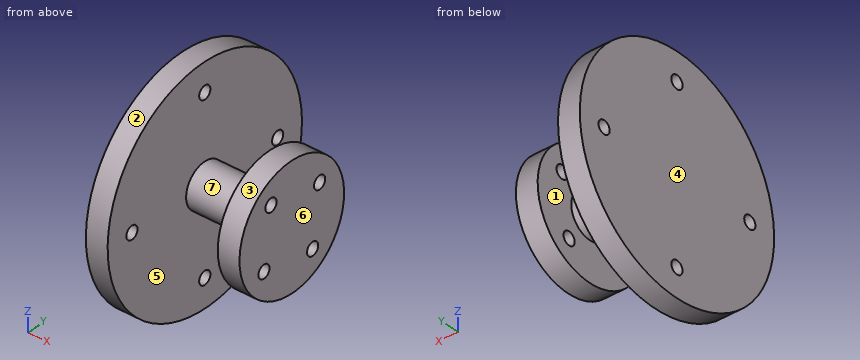
from build123d import *

# Parameters (mm, degrees)
SKETCH_2_R               = 1.5
CUT_EXTRUDE_1_DEPTH      = 45.463468151
PATTERN_CIRCULAR_1_COUNT = 4
CUT_EXTRUDE_2_REACH      = 46.463
SKETCH_3_R               = 1.5
PATTERN_CIRCULAR_2_COUNT = 4


with BuildPart() as part:
    # Sketch 1 → Revolve 1 (revolve)
    with BuildSketch(Plane.XY, mode=Mode.PRIVATE) as revolve_1_sk:
        Polygon((0, 0), (0, 26), (5, 26), (5, 5), (20, 5), (20, 14), (25, 14), (25, 0), align=None)
    revolve(revolve_1_sk.sketch.rotate(Axis((0, 0, 0), (1, 0, 0)), 90), axis=Axis((0, 0, 0), (1, 0, 0)))

    # Sketch 2 → Cut-Extrude 1 (cut, through all)
    with BuildSketch(Plane.ZY):
        with Locations((0, 19.5)):
            Circle(SKETCH_2_R)
    cut_extrude_1 = extrude(amount=-CUT_EXTRUDE_1_DEPTH, mode=Mode.SUBTRACT)

    # Pattern Circular 1: Cut-Extrude 1 ×4 about axis
    pattern_circular_1_axis = Axis((0, 0, 0), (1, 0, 0))
    for i in range(1, PATTERN_CIRCULAR_1_COUNT):
        add(cut_extrude_1.rotate(pattern_circular_1_axis, i * 360 / PATTERN_CIRCULAR_1_COUNT), mode=Mode.SUBTRACT)

    # Sketch 3 → Cut-Extrude 2 (cut, up to next)
    with BuildSketch(Plane(origin=(25, 0, 0), x_dir=(0, 0, -1), z_dir=(1, 0, 0)), mode=Mode.PRIVATE) as cut_extrude_2_sk1:
        with Locations((7.448193574, 5.569058492)):
            Circle(SKETCH_3_R)
    cut_extrude_2_tool1 = extrude(cut_extrude_2_sk1.sketch, amount=-CUT_EXTRUDE_2_REACH, mode=Mode.PRIVATE) & part.part
    cut_extrude_2 = cut_extrude_2_tool1.solids().sort_by_distance((25, 5.569058, -7.448194))[0]
    add(cut_extrude_2, mode=Mode.SUBTRACT)

    # Pattern Circular 2: Cut-Extrude 2 ×4 about axis
    pattern_circular_2_axis = Axis((0, 0, 0), (1, 0, 0))
    for i in range(1, PATTERN_CIRCULAR_2_COUNT):
        add(cut_extrude_2.rotate(pattern_circular_2_axis, i * 360 / PATTERN_CIRCULAR_2_COUNT), mode=Mode.SUBTRACT)


solid = part.part
Model file for the job. Use its own axes, mm. Face numbers are marked on the shaded views. A direction names the side the tool comes from. Round coordinates to 2 decimals unless told otherwise and drop trailing zeros. Loops run counter-clockwise (first coordinate to the right, second up) from the corner with the lowest first, then second, coordinate; pieces in that order, holes last.
1. Mould opens along X. For the marked faces 4, 5, 6 and 7 say: +X half, -X half, draft (parallel to the pull), parting line (faces both ways), or undercut.
Check values:
face 4: -X half
face 5: undercut
face 6: +X half
face 7: undercut
2. Drop flat-ended pins along their axis: P1, Ø1.8, axis at y = -5.57, z = 7.45, coming from the +X side; P2, Ø12, axis at x = 4.5, z = -15, coming from the -Y side; P3, Ø2, axis at x = 5.5, y = 1, coming from the +Z side; P4, Ø2.5, axis at y = 19.5, z = 0, coming from the +X side. Give the stop position or say it passes through.
Check values:
P1: stops at x = 5
P2: stops at y = -24.39
P3: stops at z = 26
P4: passes through
3. Band-saw the part on D-D, the plane y = -11. List the corners of the cut face in (x, z).
Check values:
outline: (0, -23.56) - (5, -23.56) - (5, 23.56) - (0, 23.56) - close; (20, -8.66) - (25, -8.66) - (25, 8.66) - (20, 8.66) - close
4. Wall check: probe 1 along Y at (x, z) = (2.25, -0.5); probe 2 along X at (y, z) = (-5.5, -10); probe 3 along X at (y, z) = (16, -2.5). Give the ranges that are in metal, low to high.
Check values:
probe 1: y = -26 to -20.91, -18.09 to 18.09, 20.91 to 26
probe 2: x = 0 to 5, 20 to 25
probe 3: x = 0 to 5
5. Tool access for the marked faces 1, 2 and 3: list every direction of +Z, -Z, +X, -X, +Y, -Y with a clear straight run to the whole face (end or side of a thin tool).
Check values:
face 1: none
face 2: +X, -X
face 3: +X
6. Band-saw the part on C-C, the plane z = 19.5. List the corners of the cut face in (x, y).
Check values:
outline: (0, -17.2) - (5, -17.2) - (5, -1.5) - (0, -1.5) - close; (0, 1.5) - (5, 1.5) - (5, 17.2) - (0, 17.2) - close
7. Band-saw the part on A-A, the plane z = 0. List the corners of the cut face in (x, y).
Check values:
outline: (0, -26) - (5, -26) - (5, -21) - (0, -21) - close; (0, -18) - (5, -18) - (5, -5) - (20, -5) - (20, -14) - (25, -14) - (25, 14) - (20, 14) - (20, 5) - (5, 5) - (5, 18) - (0, 18) - close; (0, 21) - (5, 21) - (5, 26) - (0, 26) - close
